The drawing under review shows one solid part. Ordinate dimensions are in mm from its lowest x, y, z. A direction names the side the tool comes from. Round coordinates to 2 decimals unless told otherwise and drop trailing zeros. Write each loop counter-clockwise with the first axis right and the second up, starting at its lowest first coordinate (ties: lowest second). Pieces come first, ordered by that corner, then holes. Notation, with made-up numbers: (48.5, 14.25) -> (80.5, 14.25) arc R15 cw to (80.5, 19.25) -> close; hole circle Ø8 at (-24, -30.5). An arc over 180 degrees is marked (long way). Write item = value, one per line. Start each with the question number.
Item 1: For pin 1 Ø3 at (x, y) = (6, 21.5) entering from +Z, flat-tipped, find the tip position at first contact; note if it passes through.
Item 2: Mouldability with a two-part tool opening along Y and no side actions: class the marked faces 3, 4 and 5 as released by +Y, released by -Y, zero draft, split by the parting line, or undercut.
Item 3: Add section B-B, the plane x = 8. State the section outline as (y, z) points.
Item 4: To check wall thickness, follow L1, parallel to Y at x = 49, z = 6.55; L2, parallel to Y at x = 49, z = 0.9; L3, parallel to X at y = 18, z = 1.25. State the ranges of each line that lie inside material, in increasing order.
Item 5: Add section D-D, the plane y = 19.5. State the section outline as (x, z) points.
Item 6: Add section A-A, the plane z = 7. State the section outline as (x, y) points, then the cut area to 3 significant figures.
Item 7: Machinability: for the marked faces 1 and 2, which of the approach directions +Z, -Z, +X, -X, +Y, -Y give a long, thin tool a straight path to every point of the face, cutting with its end or side? Answer none if there is none.
Item 8: Add section C-C, the plane y = 23. State the section outline as (x, z) points.
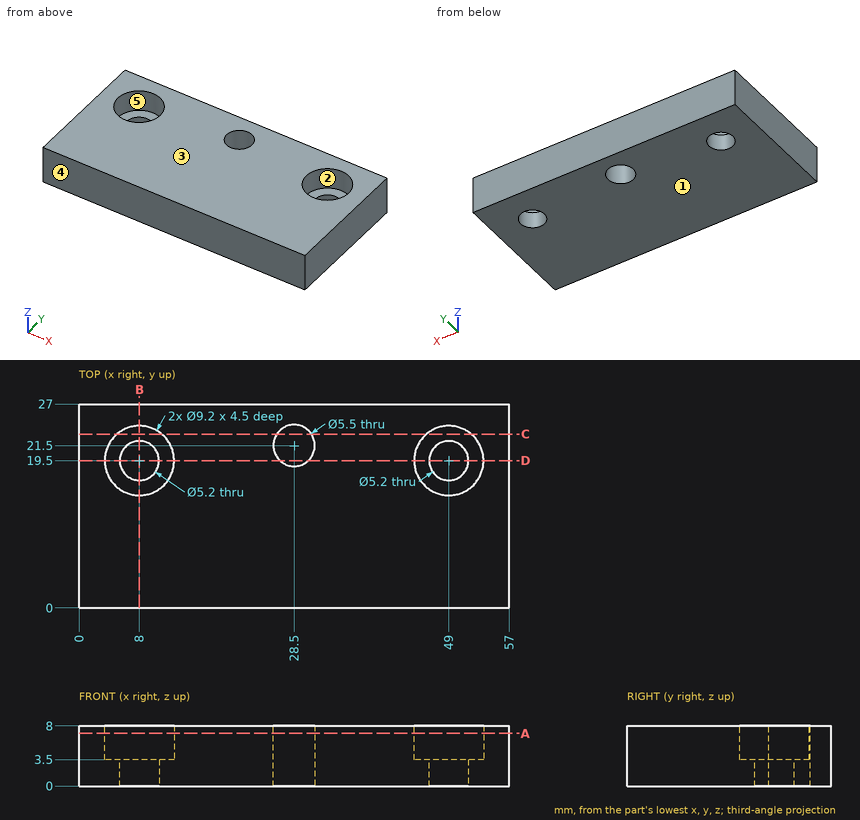
Result set:
q1.pin_1 = 3.5
q2.face_3 = zero draft
q2.face_4 = released by -Y
q2.face_5 = undercut
q3.outline = (0, 0) -> (16.9, 0) -> (16.9, 3.5) -> (14.9, 3.5) -> (14.9, 8) -> (0, 8) -> close; (22.1, 0) -> (27, 0) -> (27, 8) -> (24.1, 8) -> (24.1, 3.5) -> (22.1, 3.5) -> close
q4.L1 = 0 to 14.9, 24.1 to 27
q4.L2 = 0 to 16.9, 22.1 to 27
q4.L3 = 0 to 5.88, 10.12 to 46.88, 51.12 to 57
q5.outline = (0, 0) -> (5.4, 0) -> (5.4, 3.5) -> (3.4, 3.5) -> (3.4, 8) -> (0, 8) -> close; (10.6, 0) -> (26.61, 0) -> (26.61, 8) -> (12.6, 8) -> (12.6, 3.5) -> (10.6, 3.5) -> close; (30.39, 0) -> (46.4, 0) -> (46.4, 3.5) -> (44.4, 3.5) -> (44.4, 8) -> (30.39, 8) -> close; (51.6, 0) -> (57, 0) -> (57, 8) -> (53.6, 8) -> (53.6, 3.5) -> (51.6, 3.5) -> close
q6.outline = (0, 0) -> (57, 0) -> (57, 27) -> (0, 27) -> close; hole circle Ø9.2 at (8, 19.5); hole circle Ø5.5 at (28.5, 21.5); hole circle Ø9.2 at (49, 19.5)
q6.area = 1,380 mm²
q7.face_1 = -Z, +X, -X, +Y, -Y
q7.face_2 = +Z
q8.outline = (0, 0) -> (26.2, 0) -> (26.2, 8) -> (10.98, 8) -> (10.98, 3.5) -> (5.02, 3.5) -> (5.02, 8) -> (0, 8) -> close; (30.8, 0) -> (57, 0) -> (57, 8) -> (51.98, 8) -> (51.98, 3.5) -> (46.02, 3.5) -> (46.02, 8) -> (30.8, 8) -> close
